Geometry: final body of the model. Coordinates: model frame, mm. Give positions to 0.01 mm unless a question says otherwise; leave off trailing zeros. Write each loop counter-clockwise with the first axis right and the second up, starting at its lowest first coordinate (ties: lowest second). Pieces come first, ordered by that corner, then holes. Notation, with made-up numbers: M 24.25,-0.5 L 69.25,-0.5 A17 ccw 69.25,27.5 Z; hole C 2,2.25 d3. An arc over 180 degrees is marked long. Use a Markdown table: item, result. Add a question column.
(1) Cut plane A-A (y = 4). Output: boundary loops of the cut face in (x, z), plus the area to 3 significant figures.
(2) Draft query along Z for faces 1 (the flat face through (1, -5, 0)), 2 (the flat face through (1.12, -0.607, 2.496)), 3 (the flat face through (1.12, 0.593, -2.496)), 4 (the flat face through (0.6, -0.1, -2)). Return one class per face: released by +Z, released by -Z, zero draft, split by the parting line, or undercut.
(3) Material intervals for L1, parallel to Z at x = 0.5, y = -4.5; L2, parallel to Z at x = 0.9, y = -1.5, sorted ascending.
(4) Pin query (flat end, axial travel): pin 1 Ø0.8 at (x, z) = (1, -2.5) entering from +Y; pin 2 Ø2 at (y, z) = (-1.5, 1) entering from -X; pin 3 Ø0.8 at (x, y) = (1, -0.5) entering from +Z; pin 4 Ø0.8 at (x, z) = (1.5, -2.5) entering from -Y. Return the tip coordinate at first contact, or that it passes through.
(5) Cut plane C-C (x = 0.5). Output: boundary loops of the cut face in (y, z), plus the area to 3 significant figures.
(6) Cut plane B-B (z = -2.5). State how many separate pieces and enclosed holes the cut face has, plus the area to 3 significant figures.
```python
from build123d import *

# Parameters (mm, degrees)
SKETCH_1_W             = 4
SKETCH_1_H             = 10
EXTRUDE_1_DEPTH        = 1.5
EXTRUDE_2_DEPTH        = 1
PATTERN_LINEAR_1_COUNT = 8
PATTERN_LINEAR_1_PITCH = 1.2
MIRROR_1_COPY_1_DEPTH  = 1
MIRROR_1_COPY_2_DEPTH  = 1
MIRROR_1_COPY_3_DEPTH  = 1
MIRROR_1_COPY_4_DEPTH  = 1
MIRROR_1_COPY_5_DEPTH  = 1
MIRROR_1_COPY_6_DEPTH  = 1
MIRROR_1_COPY_7_DEPTH  = 1


with BuildPart() as part:
    # 草图1 → 凸台-拉伸1 (new body)
    with BuildSketch(Plane(origin=(0, 0, 0), x_dir=(0, 0, -1), z_dir=(1, 0, 0))):
        Rectangle(SKETCH_1_W, SKETCH_1_H)
    extrude(amount=EXTRUDE_1_DEPTH)

    # 草图2 → 凸台-拉伸2 (add)
    with BuildSketch(Plane(origin=(0, -4.7, 0), x_dir=(-1, 0, 0), z_dir=(0, -1, 0))):
        Polygon((-0.75, 2), (-1.5, 3.005587043), (-1.5, 2.65324469), (-1.012788554, 2), align=None)
    extrude_2 = extrude(amount=-EXTRUDE_2_DEPTH)

    # 阵列(线性)1: 凸台-拉伸2 ×8
    with Locations(*[(0, i * PATTERN_LINEAR_1_PITCH, 0) for i in range(1, PATTERN_LINEAR_1_COUNT)]):
        add(extrude_2)

    # 镜向1: 凸台-拉伸2 across plane
    add(extrude_2.mirror(Plane.XY))

    # 镜向1 copy 1 sketch → 镜向1 copy 1 (add)
    with BuildSketch(Plane(origin=(0, -3.5, 0), x_dir=(-1, 0, 0), z_dir=(0, -1, 0))):
        Polygon((-0.75, -2), (-1.5, -3.005587043), (-1.5, -2.65324469), (-1.012788554, -2), align=None)
    extrude(amount=-MIRROR_1_COPY_1_DEPTH)

    # 镜向1 copy 2 sketch → 镜向1 copy 2 (add)
    with BuildSketch(Plane(origin=(0, -2.3, 0), x_dir=(-1, 0, 0), z_dir=(0, -1, 0))):
        Polygon((-0.75, -2), (-1.5, -3.005587043), (-1.5, -2.65324469), (-1.012788554, -2), align=None)
    extrude(amount=-MIRROR_1_COPY_2_DEPTH)

    # 镜向1 copy 3 sketch → 镜向1 copy 3 (add)
    with BuildSketch(Plane(origin=(0, -1.1, 0), x_dir=(-1, 0, 0), z_dir=(0, -1, 0))):
        Polygon((-0.75, -2), (-1.5, -3.005587043), (-1.5, -2.65324469), (-1.012788554, -2), align=None)
    extrude(amount=-MIRROR_1_COPY_3_DEPTH)

    # 镜向1 copy 4 sketch → 镜向1 copy 4 (add)
    with BuildSketch(Plane(origin=(0, 0.1, 0), x_dir=(-1, 0, 0), z_dir=(0, -1, 0))):
        Polygon((-0.75, -2), (-1.5, -3.005587043), (-1.5, -2.65324469), (-1.012788554, -2), align=None)
    extrude(amount=-MIRROR_1_COPY_4_DEPTH)

    # 镜向1 copy 5 sketch → 镜向1 copy 5 (add)
    with BuildSketch(Plane(origin=(0, 1.3, 0), x_dir=(-1, 0, 0), z_dir=(0, -1, 0))):
        Polygon((-0.75, -2), (-1.5, -3.005587043), (-1.5, -2.65324469), (-1.012788554, -2), align=None)
    extrude(amount=-MIRROR_1_COPY_5_DEPTH)

    # 镜向1 copy 6 sketch → 镜向1 copy 6 (add)
    with BuildSketch(Plane(origin=(0, 2.5, 0), x_dir=(-1, 0, 0), z_dir=(0, -1, 0))):
        Polygon((-0.75, -2), (-1.5, -3.005587043), (-1.5, -2.65324469), (-1.012788554, -2), align=None)
    extrude(amount=-MIRROR_1_COPY_6_DEPTH)

    # 镜向1 copy 7 sketch → 镜向1 copy 7 (add)
    with BuildSketch(Plane(origin=(0, 3.7, 0), x_dir=(-1, 0, 0), z_dir=(0, -1, 0))):
        Polygon((-0.75, -2), (-1.5, -3.005587043), (-1.5, -2.65324469), (-1.012788554, -2), align=None)
    extrude(amount=-MIRROR_1_COPY_7_DEPTH)


solid = part.part
```
Answer list:
| question | item | result |
|---|---|---|
| 1 | outline | M 0,-2 L 0.75,-2 L 1.5,-3.01 L 1.5,-2.65 L 1.01,-2 L 1.5,-2 L 1.5,2 L 1.01,2 L 1.5,2.65 L 1.5,3.01 L 0.75,2 L 0,2 Z |
| 1 | area | 6.44 mm² |
| 2 | face 1 | zero draft |
| 2 | face 2 | released by +Z |
| 2 | face 3 | released by -Z |
| 2 | face 4 | undercut |
| 3 | L1 | -2 to 2 |
| 3 | L2 | -2.2 to 2.2 |
| 4 | pin 1 | y = 4.7 |
| 4 | pin 2 | x = 0 |
| 4 | pin 3 | z = 2.87 |
| 4 | pin 4 | y = -4.7 |
| 5 | outline | M -5,-2 L 5,-2 L 5,2 L -5,2 Z |
| 5 | area | 40.0 mm² |
| 6 | separate pieces | 8 |
| 6 | enclosed holes | 0 |
| 6 | area | 2.10 mm² |
